Design review of the part built by this model. Coordinates are the model's own, in mm. Face numbers are marked on the shaded views. A direction names the side the tool comes from. Coordinates: 2 decimals unless noted, no trailing zeros. Write each loop counter-clockwise with the first axis right and the second up, starting at its lowest first coordinate (ties: lowest second). Pieces come first, ordered by that corner, then holes. Notation, with made-up numbers: M 28,34 L 71,34 A20 cw 71,46 Z; hole C 10.25,-17 d11. An arc over 180 degrees is marked long. Write each question's results on one line, items separated by ' | '. Start each with the question number.
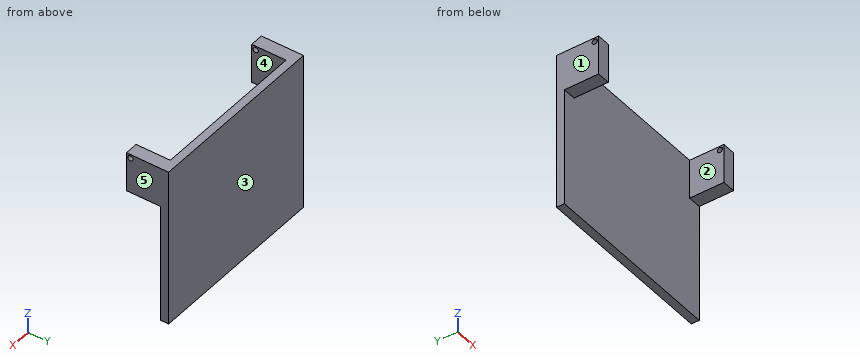
Autodesk Inventor part; units mm, degrees
ref_plane "Work Plane2" through (-23.7602, 13, -55.0885) normal (0, -1, 0) x (1, 0, 0)
ref_plane "Work Plane3" through (-70.7285, -3, -140.3642) normal (0, -1, 0) x (1, 0, 0)
ref_plane "YZ Plane" through (0, 0, 0) normal (1, 0, 0) x (0, 1, 0)
ref_plane "Work Plane1" through (-35, 0, -35) normal (0, 1, 0) x (1, 0, 0)
ref_plane "Work Plane2" through (-23.7602, 13, -55.0885) normal (0, -1, 0) x (1, 0, 0)
sketch "Sketch1" plane through (-35, 0, -35) normal (0, 1, 0) x (1, 0, 0)
  line L0 (-4, 96.5) -> (-2.5, 96.5)
  line L1 (-2.5, 96.5) -> (-2.5, 43.5)
  line L2 (-2.5, 43.5) -> (-4, 43.5)
  line L3 (-4, 43.5) -> (-4, 96.5)
  line L4 (31, 43.5) -> (31, 96.5)
  line L5 (31, 96.5) -> (32.5, 96.5)
  line L6 (32.5, 96.5) -> (32.5, 43.5)
  line L7 (32.5, 43.5) -> (31, 43.5)
  line L8 (4, 96.5) -> (4, 43.5)
  line L9 (4, 43.5) -> (2.5, 43.5)
  line L10 (2.5, 43.5) -> (2.5, 96.5)
  line L11 (2.5, 96.5) -> (4, 96.5)
  line L12 (-31, 43.5) -> (-32.5, 43.5)
  line L13 (-32.5, 43.5) -> (-32.5, 96.5)
  line L14 (-32.5, 96.5) -> (-31, 96.5)
  line L15 (-31, 96.5) -> (-31, 43.5)
  circle A0 centre (0, 0) radius 8.5
  line L16 (-35, -20) -> (-30, -20)
  line L17 (-30, -20) -> (-30, -35)
  line L18 (-30, -35) -> (30.0078, -35)
  line L19 (30.0078, -35) -> (30.0078, -20)
  line L20 (30.0078, -20) -> (35, -20)
  line L21 (35, -20) -> (35, 105)
  line L22 (35, 105) -> (-35, 105)
  line L23 (-35, 105) -> (-35, -20)
  line L24 (-35, -35) -> (35, -35)
  line L25 (35, -35) -> (35, 25)
  line L26 (35, 25) -> (-35, 25)
  line L27 (-35, 25) -> (-35, -35)
  line L28 (-4, 96.5) -> (-2.5, 96.5)
  line L29 (-2.5, 96.5) -> (-2.5, 43.5)
  line L30 (-2.5, 43.5) -> (-4, 43.5)
  line L31 (-4, 43.5) -> (-4, 96.5)
  line L32 (31, 43.5) -> (31, 96.5)
  line L33 (31, 96.5) -> (32.5, 96.5)
  line L34 (32.5, 96.5) -> (32.5, 43.5)
  line L35 (32.5, 43.5) -> (31, 43.5)
  line L36 (4, 96.5) -> (4, 43.5)
  line L37 (4, 43.5) -> (2.5, 43.5)
  line L38 (2.5, 43.5) -> (2.5, 96.5)
  line L39 (2.5, 96.5) -> (4, 96.5)
  line L40 (-31, 43.5) -> (-32.5, 43.5)
  line L41 (-32.5, 43.5) -> (-32.5, 96.5)
  line L42 (-32.5, 96.5) -> (-31, 96.5)
  line L43 (-31, 96.5) -> (-31, 43.5)
  circle A1 centre (0, 0) radius 8.5
  line L44 (-35, -20) -> (-30, -20)
  line L45 (-30, -20) -> (-30, -35)
  line L46 (-30, -35) -> (30.0078, -35)
  line L47 (30.0078, -35) -> (30.0078, -20)
  line L48 (30.0078, -20) -> (35, -20)
  line L49 (35, -20) -> (35, 105)
  line L50 (35, 105) -> (-35, 105)
  line L51 (-35, 105) -> (-35, -20)
  line L52 (-35, -35) -> (35, -35)
  line L53 (35, -35) -> (35, 25)
  line L54 (35, 25) -> (-35, 25)
  line L55 (-35, 25) -> (-35, -35)
  point P0 (35, -35)
  point P1 (35, -35)
  dimension "d0" = 60
  dimension "d3" = 60
extrude "Extrusion1" add sketch "Sketch1" along normal up to surface (13 mm away) contours A0 | L23 L26 L21 L20 L19 L18 L17 L16 | L16 L17 L24 L27 | L19 L20 L25 L24
sketch "Sketch2" plane through (-35, 0, -35) normal (0, 1, 0) x (1, 0, 0)
  line L0 (-4, 96.5) -> (-2.5, 96.5)
  line L1 (-2.5, 96.5) -> (-2.5, 43.5)
  line L2 (-2.5, 43.5) -> (-4, 43.5)
  line L3 (-4, 43.5) -> (-4, 96.5)
  line L4 (31, 43.5) -> (31, 96.5)
  line L5 (31, 96.5) -> (32.5, 96.5)
  line L6 (32.5, 96.5) -> (32.5, 43.5)
  line L7 (32.5, 43.5) -> (31, 43.5)
  line L8 (4, 96.5) -> (4, 43.5)
  line L9 (4, 43.5) -> (2.5, 43.5)
  line L10 (2.5, 43.5) -> (2.5, 96.5)
  line L11 (2.5, 96.5) -> (4, 96.5)
  line L12 (-31, 43.5) -> (-32.5, 43.5)
  line L13 (-32.5, 43.5) -> (-32.5, 96.5)
  line L14 (-32.5, 96.5) -> (-31, 96.5)
  line L15 (-31, 96.5) -> (-31, 43.5)
  circle A0 centre (0, 0) radius 8.5
  line L16 (-35, -20) -> (-30, -20)
  line L17 (-30, -20) -> (-30, -35)
  line L18 (-30, -35) -> (30.0078, -35)
  line L19 (30.0078, -35) -> (30.0078, -20)
  line L20 (30.0078, -20) -> (35, -20)
  line L21 (35, -20) -> (35, 105)
  line L22 (35, 105) -> (-35, 105)
  line L23 (-35, 105) -> (-35, -20)
  line L24 (-35, -35) -> (35, -35)
  line L25 (35, -35) -> (35, 25)
  line L26 (35, 25) -> (-35, 25)
  line L27 (-35, 25) -> (-35, -35)
  line L28 (-4, 96.5) -> (-2.5, 96.5)
  line L29 (-2.5, 96.5) -> (-2.5, 43.5)
  line L30 (-2.5, 43.5) -> (-4, 43.5)
  line L31 (-4, 43.5) -> (-4, 96.5)
  line L32 (31, 43.5) -> (31, 96.5)
  line L33 (31, 96.5) -> (32.5, 96.5)
  line L34 (32.5, 96.5) -> (32.5, 43.5)
  line L35 (32.5, 43.5) -> (31, 43.5)
  line L36 (4, 96.5) -> (4, 43.5)
  line L37 (4, 43.5) -> (2.5, 43.5)
  line L38 (2.5, 43.5) -> (2.5, 96.5)
  line L39 (2.5, 96.5) -> (4, 96.5)
  line L40 (-31, 43.5) -> (-32.5, 43.5)
  line L41 (-32.5, 43.5) -> (-32.5, 96.5)
  line L42 (-32.5, 96.5) -> (-31, 96.5)
  line L43 (-31, 96.5) -> (-31, 43.5)
  circle A1 centre (0, 0) radius 8.5
  line L44 (-35, -20) -> (-30, -20)
  line L45 (-30, -20) -> (-30, -35)
  line L46 (-30, -35) -> (30.0078, -35)
  line L47 (30.0078, -35) -> (30.0078, -20)
  line L48 (30.0078, -20) -> (35, -20)
  line L49 (35, -20) -> (35, 105)
  line L50 (35, 105) -> (-35, 105)
  line L51 (-35, 105) -> (-35, -20)
  line L52 (-35, -35) -> (35, -35)
  line L53 (35, -35) -> (35, 25)
  line L54 (35, 25) -> (-35, 25)
  line L55 (-35, 25) -> (-35, -35)
  point P0 (35, -35)
  point P1 (35, -35)
  point P2 (35, -35)
  dimension "d4" = 60
  dimension "d5" = 60
extrude "Extrusion2" cut sketch "Sketch2" against normal blind 3 from surface at 13 contours A0 | L23 L26 L21 L20 L19 L18 L17 L16 | L16 L17 L24 L27 | L19 L20 L25 L24 keep common part
sketch "Sketch3" plane through (-70, 10, 0) normal (0, -1, 0) x (1, 0, 0)
  line L0 (5, 0) -> (5, -15)
  line L1 (5, -15) -> (0, -15)
  line L2 (0, 0) -> (0, -60)
  line L3 (70, 0) -> (0, 0)
  line L4 (0, 0) -> (0, -60)
  line L5 (0, -60) -> (70, -60)
  line L6 (70, -60) -> (70, 0)
  line L7 (65.0078, -15) -> (65.0078, 0)
  line L8 (70, -15) -> (65.0078, -15)
  line L9 (70, -60) -> (70, 0)
  line L10 (0, -15) -> (5, -15)
  line L11 (5, -15) -> (5, 0)
  line L12 (5, 0) -> (0, 0)
  line L13 (0, 0) -> (0, -15)
  line L14 (65.0078, 0) -> (70, 0)
  line L15 (70, 0) -> (70, -15)
  line L16 (70, -15) -> (65.0078, -15)
  line L17 (65.0078, -15) -> (65.0078, 0)
ref_plane "Work Plane3" through (-70.7285, -3, -140.3642) normal (0, -1, 0) x (1, 0, 0)
extrude "Extrusion3" add sketch "Sketch3" along normal up to surface (13 mm away) contours L0 L1 L2 L3 | L3 L6 L8 L7
sketch "Sketch4" plane through (-70, 13, -60) normal (-1, 0, 0) x (0, 0, 1)
  line L0 (45, -16) -> (60, -16)
  line L1 (60, -13) -> (64.2426, -13) construction
  circle A0 centre (58.5, -14.5) radius 1
  dimension "d11" = 2
extrude "Extrusion4" cut sketch "Sketch4" against normal up to surface (70 mm away)
properties part number "base_3"
Item 1: We need section D-D on x = -28.5. State the section outline as (y, z) points.
Item 2: Wall thickness on L1, parallel to Y at x = -0.95, z = -1.5; L2, parallel to X at y = -1.5, z = -12; L3, parallel to Y at x = -7.5, z = -23.5: over which ranges is each line inside the solid? List them lowest first.
Item 3: For the marked faces 1 and 2, list the 3-axis set-ups (+Z, -Z, +X, -X, +Y, -Y) from which the entire face can be reached by the end or side of a thin tool; tool diameter is ignored.
Item 4: Insertion check: pin 1 Ø10 at (x, z) = (-31.5, -39) entering from -Y; pin 2 Ø6.5 at (y, z) = (3.5, -8) entering from +X; pin 3 Ø5.5 at (x, y) = (-2.5, 0.5) entering from -Z. Each pin has a flat end and moves straight along its axis. Give the tip position at first contact, or say it passes through.
Item 5: We need section C-C on z = -1.5. State the section outline as (x, y) points, then the cut area to 3 significant figures.
Item 6: We need section B-B on y = -1.5. State the section outline as (x, z) points.
Item 7: We need section A-A on y = 7.5. State the section outline as (x, z) points.
Item 8: Draft analysis for pull direction X (two halves, no side actions). For the marked faces 3, 4 and 5, state which applies: released by +X, released by -X, zero draft, split by the parting line, or undercut.
Answer:
1) outline: M 10,-60 L 13,-60 L 13,0 L 10,0 Z
2) L1: y = -3 to -2.5, -0.5 to 13 | L2: x = -70 to -65, -4.99 to 0 | L3: y = 10 to 13
3) face 1: +Z, -Z, -X, +Y, -Y | face 2: +Z, -Z, -Y
4) pin 1: stops at y = 10 | pin 2: stops at x = 0 | pin 3: stops at z = -15
5) outline: M -70,-3 L -65,-3 L -65,-2.5 L -70,-2.5 Z; M -70,-0.5 L -65,-0.5 L -65,10 L -4.99,10 L -4.99,-0.5 L 0,-0.5 L 0,13 L -70,13 Z; M -4.99,-3 L 0,-3 L 0,-2.5 L -4.99,-2.5 Z | area: 320 mm^2
6) outline: M -70,-15 L -65,-15 L -65,-2.5 L -70,-2.5 Z; M -70,-0.5 L -65,-0.5 L -65,0 L -70,0 Z; M -4.99,-15 L 0,-15 L 0,-2.5 L -4.99,-2.5 Z; M -4.99,-0.5 L 0,-0.5 L 0,0 L -4.99,0 Z
7) outline: M -70,-15 L -65,-15 L -65,0 L -70,0 Z; M -4.99,-15 L 0,-15 L 0,0 L -4.99,0 Z
8) face 3: zero draft | face 4: undercut | face 5: released by +X
